Geometry: final body of the model. Coordinates: model frame, mm. A direction names the side the tool comes from. Give positions to 0.01 mm unless a question says otherwise; leave off trailing zeros. Loops run counter-clockwise (first coordinate to the right, second up) from the corner with the lowest first, then second, coordinate; pieces in that order, holes last. Notation, with made-up numbers: M 45,70.25 L 97,70.25 A15 cw 97,85.25 Z; hole C -37,38.5 d10. An arc over 180 degrees is marked long. Put each result on its own line as item: value.
```python
from build123d import *

# Parameters (mm, degrees)
EXTRUDE_3_DEPTH          = 25
CUT_EXTRUDE_6_DEPTH      = 25
SKETCH_9_R               = 1
CUT_EXTRUDE_11_DEPTH     = 0.001
CUT_EXTRUDE_12_DEPTH     = 4
CUT_EXTRUDE_17_DEPTH     = 2
CUT_EXTRUDE_START        = 2
CUT_EXTRUDE_18_DEPTH     = 2
CUT_EXTRUDE_START_2      = 20
CUT_EXTRUDE_19_OUTLINE_R = 1.3
CUT_EXTRUDE_19_DEPTH     = 3
SKETCH_4_20_R            = 1.3
CUT_EXTRUDE_20_DEPTH     = 5


# Read off the part's stored shape, not the designer's step: 切除-拉伸19
with BuildPart() as part:
    # 草图7 → 凸台-拉伸3 (new body)
    with BuildSketch(Plane.XY):
        with BuildLine():
            Line((99.654203795, 8.309011134), (0, 0))
            ThreePointArc((0, 0), (-22.25252281, -30.663509172), (11.372685429, -48.121199083))
            Line((11.372685429, -48.121199083), (104.203277967, -10.939468499))
            ThreePointArc((104.203277967, -10.939468499), (110.217015146, 0.643574044), (99.654203795, 8.309011134))
        make_face()
    extrude(amount=EXTRUDE_3_DEPTH)

    # 草图3 → 切除-拉伸6 (cut)
    with BuildSketch(Plane.XY):
        Polygon((95.977186606, -9.138607998), (73.126313538, -14.623824499), (70.208645187, -2.469104782), (93.059518254, 3.016111719), align=None)
    extrude(amount=CUT_EXTRUDE_6_DEPTH, mode=Mode.SUBTRACT)

    # 草图9 → 切除-拉伸11 (cut)
    with BuildSketch(Plane.XY.offset(25)):
        with Locations((69.722724208, -9.013291577)):
            Circle(SKETCH_9_R)
        with Locations(Location((96.463107585, -2.594421203, 0), (0, 0, 180))):
            Circle(SKETCH_9_R)
    extrude(amount=-CUT_EXTRUDE_11_DEPTH, mode=Mode.SUBTRACT)

    # 草图3<11> → 切除-拉伸12 (cut)
    with BuildSketch(Plane.XY):
        Polygon((72.842644051, -13.442085282), (67.980756164, -14.609152622), (65.701162058, -5.112587525), (70.563049944, -3.945520185), align=None)
    extrude(amount=CUT_EXTRUDE_12_DEPTH, mode=Mode.SUBTRACT)

    # Sketch 3D_5 → 切除-拉伸17 (cut)
    with BuildSketch(Plane(origin=(10.444215818, -27.693919668, 25), x_dir=(-0.9953297932940416, 0.09653290931718772, 0), z_dir=(0, 0, -1))):
        with BuildLine():
            Line((0, 0), (-18.453401997, 8.947839585))
            ThreePointArc((-18.453401997, 8.947839585), (-18.48417706, 8.964108788), (-18.513745535, 8.982479872))
            ThreePointArc((-18.513745535, 8.982479872), (-19.45567303, 12.165265617), (-16.502248474, 13.680071182))
            Line((-16.502248474, 13.680071182), (3.235389304, 9.299601756))
            ThreePointArc((3.235389304, 9.299601756), (3.842109592, 9.12676054), (4.424199035, 8.883541558))
            Line((4.424199035, 8.883541558), (22.585849479, 0))
            ThreePointArc((22.585849479, 0), (23.950111663, -3.025911631), (21.229027313, -4.926714742))
            ThreePointArc((21.229027313, -4.926714742), (21.194456039, -4.922638166), (21.160252198, -4.916166022))
            Line((21.160252198, -4.916166022), (1.154440034, -0.404031474))
            ThreePointArc((1.154440034, -0.404031474), (0.56560873, -0.235192692), (0, 0))
        make_face()
    extrude(amount=CUT_EXTRUDE_17_DEPTH, mode=Mode.SUBTRACT)

    # 草图4<19> → 切除-拉伸18 (cut)
    with BuildSketch(Plane.XY.offset(CUT_EXTRUDE_START)):
        with BuildLine():
            Line((29.675197601, -20.569228925), (10.444215818, -27.693919668))
            ThreePointArc((10.444215818, -27.693919668), (9.858544762, -27.873414105), (9.256164924, -27.984622777))
            Line((9.256164924, -27.984622777), (-11.091785437, -30.544465472))
            ThreePointArc((-11.091785437, -30.544465472), (-11.126454314, -30.547605594), (-11.161257657, -30.548325866))
            ThreePointArc((-11.161257657, -30.548325866), (-13.686143926, -28.393725709), (-12.036153076, -25.513641909))
            Line((-12.036153076, -25.513641909), (6.898232818, -18.424785281))
            ThreePointArc((6.898232818, -18.424785281), (7.50108242, -18.23889297), (8.121654063, -18.125427433))
            Line((8.121654063, -18.125427433), (28.189972451, -15.670747301))
            ThreePointArc((28.189972451, -15.670747301), (30.983375316, -17.463581076), (29.738603249, -20.540575553))
            ThreePointArc((29.738603249, -20.540575553), (29.707399451, -20.556006509), (29.675197601, -20.569228925))
        make_face()
    extrude(amount=-CUT_EXTRUDE_18_DEPTH, mode=Mode.SUBTRACT)

    # 切除-拉伸19 outline → 切除-拉伸19 (cut)
    with BuildSketch(Plane.XY.offset(CUT_EXTRUDE_START_2)):
        with Locations((27.642515471, -18.415074729)):
            Circle(CUT_EXTRUDE_19_OUTLINE_R)
        with Locations((23.660004397, -19.389551795)):
            Circle(CUT_EXTRUDE_19_OUTLINE_R)
        with Locations((19.947149108, -20.298047028)):
            Circle(CUT_EXTRUDE_19_OUTLINE_R)
        with Locations((-2.588035502, -25.812161156)):
            Circle(CUT_EXTRUDE_19_OUTLINE_R)
        with Locations((-6.300890791, -26.72065639)):
            Circle(CUT_EXTRUDE_19_OUTLINE_R)
        with Locations((-10.283401864, -27.695133455)):
            Circle(CUT_EXTRUDE_19_OUTLINE_R)
    extrude(amount=CUT_EXTRUDE_19_DEPTH, mode=Mode.SUBTRACT)

    # 草图4<20> → 切除-拉伸20 (cut)
    with BuildSketch(Plane.XY):
        with Locations(Location((-2.588035502, -25.812161156, 0), (0, 0, 180))):
            Circle(SKETCH_4_20_R)
        with Locations(Location((27.642515471, -18.415074729, 0), (0, 0, 180))):
            Circle(SKETCH_4_20_R)
        with Locations(Location((23.660004397, -19.389551795, 0), (0, 0, 180))):
            Circle(SKETCH_4_20_R)
        with Locations(Location((19.947149108, -20.298047028, 0), (0, 0, 180))):
            Circle(SKETCH_4_20_R)
        with Locations(Location((-6.300890791, -26.72065639, 0), (0, 0, 180))):
            Circle(SKETCH_4_20_R)
        with Locations(Location((-10.283401864, -27.695133455, 0), (0, 0, 180))):
            Circle(SKETCH_4_20_R)
    extrude(amount=CUT_EXTRUDE_20_DEPTH, mode=Mode.SUBTRACT)


solid = part.part
```
Item 1: Line query: probe 1 along X at (y, z) = (-19.5, 2.75); probe 2 along X at (y, z) = (-2.5, 2.5); probe 3 along Y at (x, z) = (85.5, 10.75). Output: solid intervals per line, ascending. Write a range as [from, to].
Output values:
probe 1: [-22.33, 18.92], [20.97, 22.36], [24.96, 26.93], [28.36, 82.83]
probe 2: [-9, 70.22], [94.38, 110.45]
probe 3: [-18.43, -11.65], [1.2, 7.13]
Item 2: Set-up query: faces 1 (the cylindrical face through (20.905, -21.177, 3.479)), 2 (the cylindrical face through (-10.453, -26.406, 21.479)), 3 (the flat face through (81.474, 0.235, 12.325)). Return all of +Z, -Z, +X, -X, +Y, -Y with unobstructed straight access to the full face (end or side cutting, diameter ignored); none if empty.
Output values:
face 1: -Z
face 2: +Z
face 3: +Z, -Z
Item 3: Section B-B on y = -32.5. Output: boundary loops of the cut face in (x, z).
Output values:
outline: M -21.74,0 L 50.37,0 L 50.37,25 L -21.74,25 Z
Item 4: Section A-A on z = 16.5. Output: boundary loops of the cut face in (x, y), then the cut area to 3 significant figures.
Output values:
outline: M 0,0 A25 ccw long 11.37,-48.12 L 104.2,-10.94 A10 ccw 99.65,8.31 Z; hole M 70.21,-2.47 L 73.13,-14.62 L 95.98,-9.14 L 93.06,3.02 Z
area: 4,420 mm²
Item 5: Pin query (flat end, axial travel): pin 1 Ø3 at (y, z) = (-23, 3) entering from +X; pin 2 Ø2 at (x, y) = (27, -19) entering from +Z; pin 3 Ø1.6 at (x, y) = (-2.59, -25.81) entering from -Z. Return the tip coordinate at first contact, or that it passes through.
Output values:
pin 1: x = 77.84
pin 2: z = 23
pin 3: z = 5
Item 6: Section C-C on x = 53. Output: boundary loops of the cut face in (y, z).
Output values:
outline: M -31.45,0 L 4.42,0 L 4.42,25 L -31.45,25 Z
Item 7: Mould query, pull axis Y, two halves, no side actions, for faces 4 (the flat face through (50.525, 4.213, 12.325)), 5 (the flat face through (28, -14, 0)), 6 (the cylindrical face through (-10.88, -26.54, 3.48)), 7 (the flat face through (19.93, -24.18, 24.01)). Classes: pulls with the +Y half, pulls with the -Y half, needs draft (parallel to the pull), parting line crosses it, or undercut.
Output values:
face 4: pulls with the +Y half
face 5: needs draft
face 6: undercut
face 7: undercut
